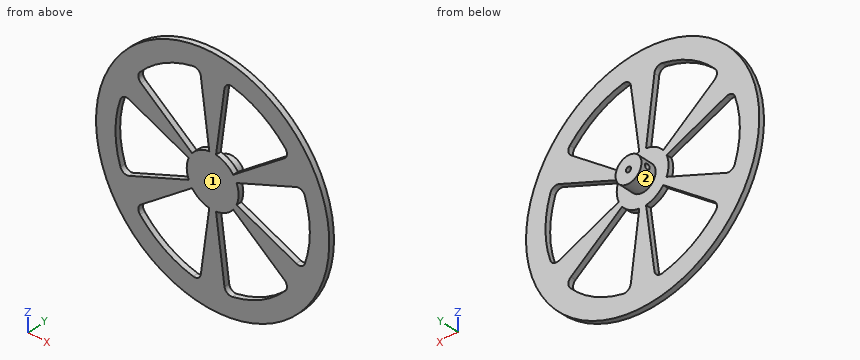
from build123d import *

# Parameters (mm, degrees)
SKETCH_1_R               = 90
EXTRUDE_1_DEPTH          = 4
CUT_EXTRUDE_1_DEPTH      = 128.342059038
PATTERN_CIRCULAR_1_COUNT = 6
SKETCH_6_R               = 10
EXTRUDE_2_DEPTH          = 12
SKETCH_7_R               = 2
CUT_EXTRUDE_2_DEPTH      = 12
FILLET_1_R               = 5
FILLET_2_R               = 5
SKETCH_9_R               = 2
CUT_EXTRUDE_3_DEPTH      = 10


with BuildPart() as part:
    # Sketch 1 → Extrude 1 (new body)
    with BuildSketch(Plane(origin=(0, 0, 0), x_dir=(1, 0, 0), z_dir=(0, 1, 0))):
        with Locations(Location((0, 0, 0), (0, 0, 270))):
            Circle(SKETCH_1_R)
    extrude(amount=EXTRUDE_1_DEPTH)

    # Sketch 2 → Cut-Extrude 1 (cut, through all)
    with BuildSketch(Plane(origin=(0, 4, 0), x_dir=(1, 0, 0), z_dir=(0, 1, 0))):
        with BuildLine():
            ThreePointArc((-15.867066806, 12.17522858), (-10, 17.320508076), (-2.610523844, 19.828897227))
            Line((-2.610523844, 19.828897227), (-9.789464417, 74.358364603))
            ThreePointArc((-9.789464417, 74.358364603), (-37.5, 64.951905284), (-59.501500522, 45.657107176))
            Line((-59.501500522, 45.657107176), (-15.867066806, 12.17522858))
        make_face()
    cut_extrude_1 = extrude(amount=-CUT_EXTRUDE_1_DEPTH, mode=Mode.SUBTRACT)

    # Pattern Circular 1: Cut-Extrude 1 ×6 about axis
    pattern_circular_1_axis = Axis((0, 0, 0), (0, 1, 0))
    for i in range(1, PATTERN_CIRCULAR_1_COUNT):
        add(cut_extrude_1.rotate(pattern_circular_1_axis, i * 360 / PATTERN_CIRCULAR_1_COUNT), mode=Mode.SUBTRACT)

    # Sketch 6 → Extrude 2 (add)
    with BuildSketch(Plane(origin=(0, 4, 0), x_dir=(1, 0, 0), z_dir=(0, 1, 0))):
        with Locations(Location((0, 0, 0), (0, 0, 270))):
            Circle(SKETCH_6_R)
    extrude(amount=EXTRUDE_2_DEPTH)

    # Sketch 7 → Cut-Extrude 2 (cut)
    with BuildSketch(Plane(origin=(0, 16, 0), x_dir=(1, 0, 0), z_dir=(0, 1, 0))):
        with Locations(Location((0, 0, 0), (0, 0, 270))):
            Circle(SKETCH_7_R)
    extrude(amount=-CUT_EXTRUDE_2_DEPTH, mode=Mode.SUBTRACT)

    # Fillet 1
    fillet_1_edges = [part.edges().sort_by_distance(p)[0] for p in [
        (9.789464417, 2, 74.358364603),
    ]]
    fillet(fillet_1_edges, radius=FILLET_1_R)

    # Fillet 2
    fillet_2_edges = [part.edges().sort_by_distance(p)[0] for p in [
        (-59.501500522, 2, -45.657107176),
        (-59.501500522, 2, 45.657107176),
        (-9.789464417, 2, 74.358364603),
        (59.501500522, 2, 45.657107176),
        (59.501500522, 2, -45.657107176),
        (9.789464417, 2, -74.358364603),
        (69.290964938, 2, 28.701257427),
        (69.290964938, 2, -28.701257427),
        (-69.290964938, 2, -28.701257427),
        (-69.290964938, 2, 28.701257427),
        (-9.789464417, 2, -74.358364603),
    ]]
    fillet(fillet_2_edges, radius=FILLET_2_R)

    # Sketch 9 → Cut-Extrude 3 (cut)
    with BuildSketch(Plane(origin=(0, 0, 0), x_dir=(0, 0, -1), z_dir=(1, 0, 0))):
        with Locations((0, 11)):
            Circle(SKETCH_9_R)
    extrude(amount=-CUT_EXTRUDE_3_DEPTH, mode=Mode.SUBTRACT)


solid = part.part
For this review, take the finished solid that the model builds, in its own axes (mm). Face numbers are marked on the shaded views. Round coordinates to 2 decimals unless told otherwise and drop trailing zeros. Loops run counter-clockwise (first coordinate to the right, second up) from the corner with the lowest first, then second, coordinate; pieces in that order, holes last. Notation, with made-up numbers: (47.5, 18.25) - (66.5, 18.25) arc R38 cw to (66.5, 57.25) - close; hole circle Ø2 at (-34, 25). An arc over 180 degrees is marked (long way). One line per item, written item: value. Start each with the question number.
Item 1: Clearance check with flat-ended pins moving along their axes: pin 1 Ø1.2 at (x, z) = (0.5, 0) entering from +Y; pin 2 Ø2 at (x, y) = (-40, 3) entering from -Z; pin 3 Ø6.5 at (y, z) = (11, 0) entering from +X. State where each tip first meets the part, or that it passes through.
Item 2: Take a section at A-A (z = 60). Give the boundary of the cut face in (x, y).
Item 3: Take a section at D-D (x = -51). Give the boundary of the cut face in (y, z).
Item 4: For L1, parallel to Z at x = 16.5, y = 1.75; L2, parallel to X at y = 13.75, z = 0; L3, parallel to Y at x = 64, z = -58, list the stretches that pass through material, from the lowest coordinate up.
Item 5: The part is to be moulded in two halves that separate along Z. For the marked faces 1 and 2, say which applies: +Z half, -Z half, draft (parallel to the pull), parting line (faces both ways), or undercut.
Item 6: Take a section at B-B (x = -30.5). Give the boundary of the cut face in (y, z), plus the area to 3 significant figures.
Item 7: Take a section at C-C (x = 61.5). Give the boundary of the cut face in (y, z).
Answer below:
1. pin 1: stops at y = 4
1. pin 2: stops at z = -81.11
1. pin 3: stops at x = 10
2. outline: (-67.08, 0) - (-45, 0) - (-45, 4) - (-67.08, 4) - close; (-7.9, 0) - (7.9, 0) - (7.9, 4) - (-7.9, 4) - close; (45, 0) - (67.08, 0) - (67.08, 4) - (45, 4) - close
3. outline: (0, -74.16) - (4, -74.16) - (4, -54.99) - (0, -54.99) - close; (0, -39.13) - (4, -39.13) - (4, -21.12) - (0, -21.12) - close; (0, 21.12) - (4, 21.12) - (4, 39.13) - (0, 39.13) - close; (0, 54.99) - (4, 54.99) - (4, 74.16) - (0, 74.16) - close
4. L1: z = -88.47 to -73.16, -12.66 to 12.66, 73.16 to 88.47
4. L2: x = -10 to -2, 2 to 10
4. L3: y = 0 to 4
5. face 1: draft
5. face 2: parting line
6. outline: (0, -84.67) - (4, -84.67) - (4, -68.52) - (0, -68.52) - close; (0, -23.4) - (4, -23.4) - (4, -12.63) - (0, -12.63) - close; (0, 12.63) - (4, 12.63) - (4, 23.4) - (0, 23.4) - close; (0, 68.52) - (4, 68.52) - (4, 84.67) - (0, 84.67) - close
6. area: 215 mm2
7. outline: (0, -65.71) - (4, -65.71) - (4, -25.47) - (0, -25.47) - close; (0, 25.47) - (4, 25.47) - (4, 65.71) - (0, 65.71) - close
